Input: part model. Units: mm. Frame: model coordinates. A direction names the side the tool comes from. Coordinates: 2 decimals unless noted, no trailing zeros. Loops run counter-clockwise (first coordinate to the right, second up) from the corner with the lowest first, then second, coordinate; pieces in that order, holes last. Notation, with made-up numbers: (51.5, 10) -> (63.5, 10) arc R30 ccw to (63.5, 41) -> close; hole circle Ø8 at (23.5, 42). An arc over 180 degrees is marked (long way). Put each result on its own line as item: value. Start each with the question number.
1) Cut plane A-A (y = -0.75). Return the cut outline in (x, z).
2) Material intervals for L1, parallel to Z at x = 0, y = -0.2 (3 decimals); L2, parallel to X at y = -0.3, z = 0 (3 decimals); L3, parallel to Z at x = -1, y = -1.65, sorted ascending.
3) Cut plane B-B (x = 2.9). Return the cut outline in (y, z).
4) Contact query for flat-ended pins moving along their axis: P1, Ø0.5, axis at x = -1, y = -1.5, coming from the -Z side; P2, Ø1.9, axis at y = -1.5, z = -0.5, coming from the -X side; P3, Ø1, axis at x = 1.5, z = 0.5, coming from the -Y side. Output: stop coordinate, or through.
5) Cut plane C-C (z = -1.45). Return the cut outline in (x, y).
6) Set-up query: faces 1 (the flat face through (-0.74, 1.048, 1.006)), 2 (the flat face through (-1.5, -1, 0)), 3 (the flat face through (-0.37, -1.36, 0.62)), 4 (the flat face through (-0.8, 1, -1)), 5 (the cylindrical face through (1.05, 1.05, -0.02)). Return all of +Z, -Z, +X, -X, +Y, -Y with unobstructed straight access to the full face (end or side cutting, diameter ignored); none if empty.
from build123d import *

# Parameters (mm, degrees)
BOSS_EXTRUDE1_DEPTH     = 2.125
SKETCH4_R               = 0.35
THROUGH_HOLES_DEPTH     = 4.445014514
FILLET1_R               = 0.125
SKETCH5_R               = 0.125
BOSS_EXTRUDE2_DEPTH     = 0.5
SKETCH8_R               = 0.46
CUT_EXTRUDE1_DEPTH      = 5.582575695
CUT_EXTRUDE2_DEPTH      = 5.367851302
CUT_EXTRUDE2_DEPTH_BACK = 5.367851302
SKETCH9_W               = 1.465031661
SKETCH9_H               = 4
BOSS_EXTRUDE3_DEPTH     = 1.75
FILLET2_R               = 0.1


with BuildPart() as part:
    # Sketch3 → Boss-Extrude1 (new body)
    with BuildSketch(Plane(origin=(0, 0, 0), x_dir=(1, 0, 0), z_dir=(0, 1, 0))):
        with BuildLine():
            Line((-2.5, 0.9), (-2, 0.93))
            Line((-2, 0.93), (-2, 0.56))
            Line((-2, 0.56), (-1.5, 0.56))
            Line((-1.5, 0.56), (-1.5, 0.96))
            Line((-1.5, 0.96), (0, 1.05))
            ThreePointArc((0, 1.05), (1.05, 0), (0, -1.05))
            Line((0, -1.05), (-1.5, -0.96))
            Line((-1.5, -0.96), (-1.5, -0.56))
            Line((-1.5, -0.56), (-2, -0.56))
            Line((-2, -0.56), (-2, -0.93))
            Line((-2, -0.93), (-2.5, -0.9))
            Line((-2.5, -0.9), (-2.5, 0.9))
        make_face()
    extrude(amount=BOSS_EXTRUDE1_DEPTH)

    # Sketch4 → Through Holes (cut, through all)
    with BuildSketch(Plane(origin=(0, 2.125, 0), x_dir=(1, 0, 0), z_dir=(0, 1, 0))):
        with Locations(Location((0, 0, 0), (0, 0, 270))):
            Circle(SKETCH4_R)
    extrude(amount=-THROUGH_HOLES_DEPTH, mode=Mode.SUBTRACT)

    # Fillet1
    fillet1_edges = [part.edges().sort_by_distance(p)[0] for p in [
        (-2, 1.0625, -0.56),
        (-1.5, 1.0625, -0.56),
        (-1.5, 1.0625, 0.56),
        (-2, 1.0625, 0.56),
    ]]
    fillet(fillet1_edges, radius=FILLET1_R)

    # Sketch5 → Boss-Extrude2 (add)
    with BuildSketch(Plane(origin=(0, 0, 0), x_dir=(1, 0, 0), z_dir=(0, 1, 0))):
        Polygon((-2.25, -2), (1.75, -2), (3.25, -2), (3.25, 2), (1.75, 2), (-2.25, 2), align=None)
        with Locations(Location((0, 0, 0), (0, 0, 270))):
            Circle(SKETCH5_R, mode=Mode.SUBTRACT)
    extrude(amount=-BOSS_EXTRUDE2_DEPTH)

    # Sketch8 → Cut-Extrude1 (cut, through all)
    with BuildSketch(Plane(origin=(0.7, 2.1, 0), x_dir=(0.948683298050514, -0.3162277660168378, 0), z_dir=(0.3162277660168378, 0.948683298050514, 0))):
        with Locations((1.987936011, 0)):
            Circle(SKETCH8_R)
    extrude(amount=-CUT_EXTRUDE1_DEPTH, mode=Mode.SUBTRACT)

    # Sketch9 → Cut-Extrude2 (cut, two sides: drawn at the far end of the back side and taken through both)
    with BuildSketch(Plane.XZ.offset(-CUT_EXTRUDE2_DEPTH_BACK)):
        with Locations((-2.982515831, 0)):
            Rectangle(SKETCH9_W, SKETCH9_H)
    extrude(amount=CUT_EXTRUDE2_DEPTH + CUT_EXTRUDE2_DEPTH_BACK, mode=Mode.SUBTRACT)

    # Sketch10 → Boss-Extrude3 (add)
    with BuildSketch(Plane.XZ.offset(0.5)):
        Polygon((-1.5, 1.25), (-1.5, -1.25), (-0.75, -1.25), (0, 0), (-0.75, 1.25), align=None)
    extrude(amount=BOSS_EXTRUDE3_DEPTH)

    # Fillet2
    fillet2_edges = [part.edges().sort_by_distance(p)[0] for p in [
        (-0.75, -1.375, 1.25),
        (-1.5, -1.375, 1.25),
        (-1.5, -1.375, -1.25),
        (-0.75, -1.375, -1.25),
        (0, -1.375, 0),
    ]]
    fillet(fillet2_edges, radius=FILLET2_R)


solid = part.part
Results found:
1. outline: (-1.5, -1.15) arc R0.1 ccw to (-1.4, -1.25) -> (-0.81, -1.25) arc R0.1 ccw to (-0.72, -1.2) -> (-0.03, -0.05) arc R0.1 ccw to (-0.03, 0.05) -> (-0.72, 1.2) arc R0.1 ccw to (-0.81, 1.25) -> (-1.4, 1.25) arc R0.1 ccw to (-1.5, 1.15) -> close
2. L1: z = -2 to -0.125, 0.125 to 2
2. L2: x = -2.25 to -0.125, 0.125 to 1.511, 2.48 to 3.25
2. L3: z = -1.25 to 1.25
3. outline: (-0.5, -2) -> (0, -2) -> (0, 2) -> (-0.5, 2) -> close
4. P1: stops at z = -1.25
4. P2: stops at x = -1.5
4. P3: stops at y = -0.5
5. outline: (-2.25, -0.5) -> (3.25, -0.5) -> (3.25, 0) -> (-2.25, 0) -> close
6. face 1: +Z, -X, +Y
6. face 2: +Z, -Z, -X, -Y
6. face 3: +Z, +X, -Y
6. face 4: -Z, -X, +Y
6. face 5: +X, +Y
